Here's the drawing with two shaded views (mm, measured from the low corner). I have some questions. A direction names the side the tool comes from. Give positions to 0.01 mm unless a question says otherwise; leave off trailing zeros. Order: outer loops, then holes, each group sorted by start corner. A loop starts at its lowest first (then second) coordinate and runs counter-clockwise, first axis right, second up. Notation, with made-up numbers: M -29.5,29 L -8.5,29 A21 ccw -8.5,35 Z; hole C 20.25,74.25 d7. An arc over 180 degrees is marked long. Use a Markdown table: item, result. Add a question column.
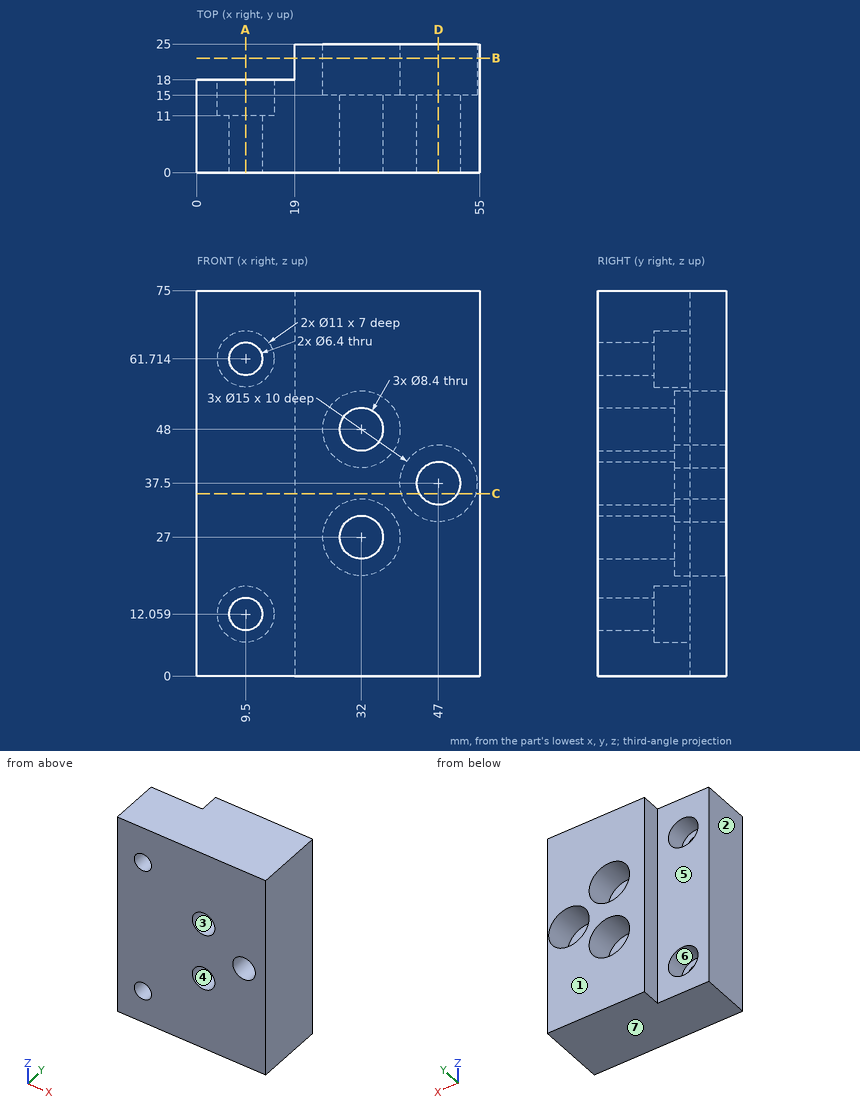
1) Suppose I cut it at A-A on x = 9.5. Please give me the cut outline in (y, z).
2) Suppose I cut it at B-B on y = 22.25. Please give me the cut outline in (x, z), and give its area (3 significant figures).
3) We'd pull the mould along X, two halves only. Please class the marked faces 1, 2, 3 and 4: pulls with the +X half, pulls with the -X half, needs draft (parallel to the pull), parting line crosses it, or undercut.
4) Suppose I cut it at C-C on z = 35.5. Please give me the cut outline in (x, y).
5) Suppose I cut it at D-D on x = 47. Please give me the cut outline in (y, z), and give its area (3 significant figures).
6) For the marked faces 5, 6 and 7, which set-ups out of +Z, -Z, +X, -X, +Y, -Y let a thin tool reach every point of the face, with its end or its side?
7) Please list where these lines run through material, in increasing order: line 1 (Z direction, x = 9.5, y = 14.25); line 2 (Z direction, x = 32, y = 21); line 3 (Z direction, x = 47, y = 19). Write a range as from..to.
8) For pin 1 (2 mm diameter, centred on y = 22, z = 28, fed in from -X); pin 2 (1 mm diameter, centred on x = 29.5, z = 42.5, fed in from +Y); pin 3 (9 mm diameter, centred on x = 9.5, z = 61.714, fed in from +Y); pin 4 (6.5 mm diameter, centred on x = 32, z = 27, fed in from +Y), each with a flat end and sliding along its axis, tell me the tip position at first contact or that it passes through.
Values found:
| question | item | result |
|---|---|---|
| 1 | outline | M 0,0 L 18,0 L 18,6.56 L 11,6.56 L 11,8.86 L 0,8.86 Z; M 0,15.26 L 11,15.26 L 11,17.56 L 18,17.56 L 18,56.21 L 11,56.21 L 11,58.51 L 0,58.51 Z; M 0,64.91 L 11,64.91 L 11,67.21 L 18,67.21 L 18,75 L 0,75 Z |
| 2 | outline | M 19,0 L 55,0 L 55,75 L 19,75 Z; hole C 32,27 d15; hole C 32,48 d15; hole C 47,37.5 d15 |
| 2 | area | 2,170 mm^2 |
| 3 | face 1 | needs draft |
| 3 | face 2 | pulls with the -X half |
| 3 | face 3 | undercut |
| 3 | face 4 | undercut |
| 4 | outline | M 0,0 L 43.31,0 L 43.31,15 L 39.77,15 L 39.77,25 L 19,25 L 19,18 L 0,18 Z; M 50.69,0 L 55,0 L 55,25 L 54.23,25 L 54.23,15 L 50.69,15 Z |
| 5 | outline | M 0,0 L 25,0 L 25,30 L 15,30 L 15,33.3 L 0,33.3 Z; M 0,41.7 L 15,41.7 L 15,45 L 25,45 L 25,75 L 0,75 Z |
| 5 | area | 1,600 mm^2 |
| 6 | face 5 | +Z, -Z, -X, +Y |
| 6 | face 6 | +Y |
| 6 | face 7 | -Z, +X, -X, +Y, -Y |
| 7 | line 1 | z = 0..6.56, 17.56..56.21, 67.21..75 |
| 7 | line 2 | z = 0..19.5, 34.5..40.5, 55.5..75 |
| 7 | line 3 | z = 0..30, 45..75 |
| 8 | pin 1 | stops at x = 19 |
| 8 | pin 2 | stops at y = 15 |
| 8 | pin 3 | stops at y = 11 |
| 8 | pin 4 | passes through |
